Solid Edge part; units mm, degrees
sketch "Sketch1" plane through (0, 0, 0) normal (0, 0, 1) x (1, 0, 0)
  circle A0 centre (0, 0) radius 2.5
extrude "Ajout_matière_1" add sketch "Sketch1" along normal blind 20
sketch "Sketch2" plane through (0, 0, 20) normal (0, 0, 1) x (1, 0, 0)
  circle A0 centre (0, 0) radius 1.55
extrude "Ajout_matière_2" add sketch "Sketch2" along normal blind 3
mirror "Mirror1" about plane through (0, 0, 0) normal (0, 0, 1) of "Ajout_matière_1", "Ajout_matière_2"
properties material "Acier S235"
Could you check a few things on this model? Use its own coordinates, in mm. A direction names the side the tool comes from. Coordinates: 2 decimals unless noted, no trailing zeros. Order: outer loops, then holes, each group sorted by start corner. A loop starts at its lowest first (then second) coordinate and runs counter-clockwise, first axis right, second up. Notation, with made-up numbers: M 65.5,-34.75 L 98.5,-34.75 A12 cw 98.5,-21.75 Z; hole C -2.5,50.5 d8. An arc over 180 degrees is marked long. Use a Markdown table: item, result. Add a question column.
Q1. I want a section at C-C on z = 8. List the corners of the cut face in (x, y) for me.
Q2. I want a section at A-A on y = 0. List the corners of the cut face in (x, z) for me, then the cut area to 3 significant figures.
Q3. Which directions (+Z, -Z, +X, -X, +Y, -Y) give clear straight access to the entire face, cutting with the end or side of a thin tool? Please do faces 1 (the flat face through (0, 0, 23)), 2 (the cylindrical face through (0.715, -1.375, -21.479)), 3 (the cylindrical face through (0.715, 1.375, 21.479)).
Q4. If I drill on L1, parallel to Y at x = 0.2, z = 7; L2, parallel to Z at x = 1.15, y = -1.9; L3, parallel to X at y = 1.05, z = 21.5, over which ranges is the centre line in solid material (lowest first)?
Q5. I want a section at D-D on x = -2.05. List the corners of the cut face in (y, z) for me, then the cut area to 3 significant figures.
Q6. I'm going to push a flat-ended pin straight in: pin 1 (3 mm diameter, centred on y = 1.5, z = 4, fed in from -X). Where does the tip first touch, or does it pass through?
Checked values:
| question | item | result |
|---|---|---|
| 1 | outline | C 0,0 d5 |
| 2 | outline | M -2.5,-20 L -1.55,-20 L -1.55,-23 L 1.55,-23 L 1.55,-20 L 2.5,-20 L 2.5,20 L 1.55,20 L 1.55,23 L -1.55,23 L -1.55,20 L -2.5,20 Z |
| 2 | area | 219 mm² |
| 3 | face 1 | +Z, +X, -X, +Y, -Y |
| 3 | face 2 | -Z |
| 3 | face 3 | +Z |
| 4 | L1 | -2.49 to 2.49 |
| 4 | L2 | -20 to 20 |
| 4 | L3 | -1.14 to 1.14 |
| 5 | outline | M -1.43,-20 L 1.43,-20 L 1.43,20 L -1.43,20 Z |
| 5 | area | 114 mm² |
| 6 | pin 1 | x = -2.5 |
